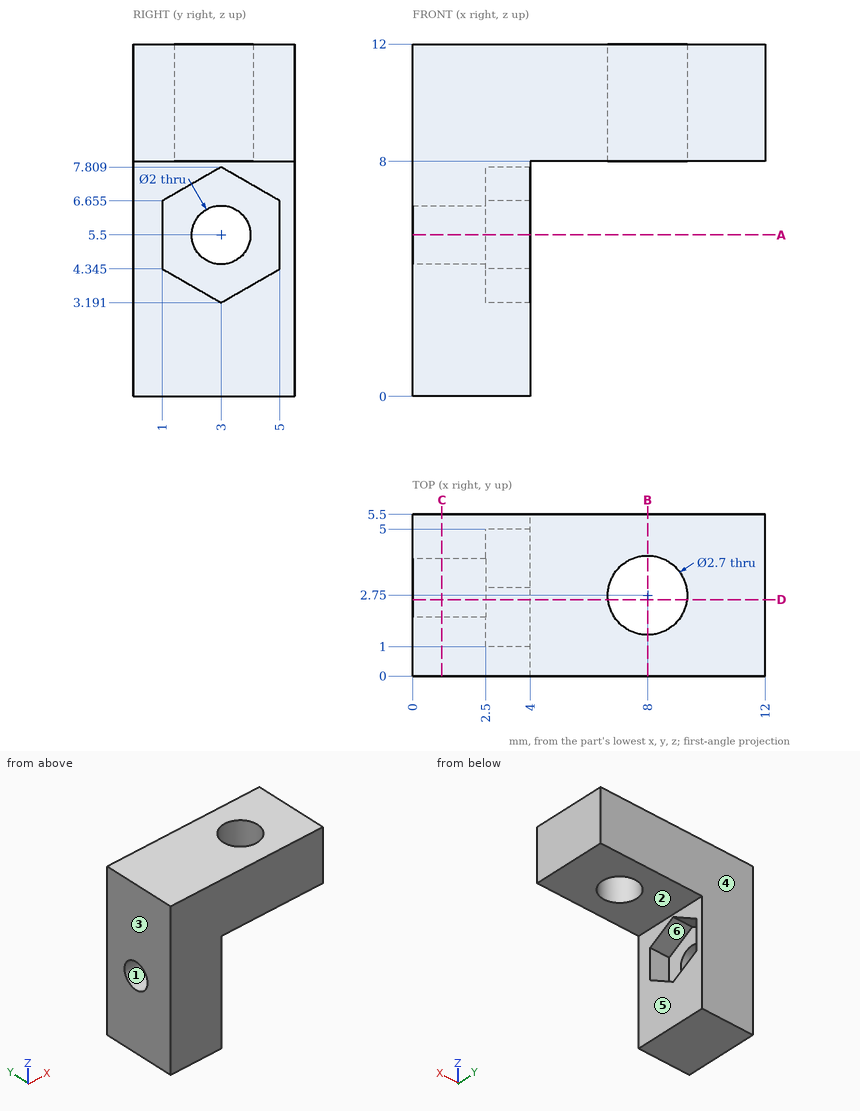
Geometry check sheet. Reference: drawing and pictorial views, mm from the part's lowest x, y, z. A direction names the side the tool comes from. Give positions to 0.01 mm unless a question says otherwise; leave off trailing zeros. Order: outer loops, then holes, each group sorted by start corner. A loop starts at its lowest first (then second) coordinate and runs counter-clockwise, first axis right, second up. Notation, with made-up numbers: M 86,25.5 L 102,25.5 A23 cw 102,48.5 Z; hole C 1.25,84 d3. An arc over 180 degrees is marked long. Use one line per item in the form item = value. Start each with the question number.
Q1. Section check B-B (x = 8). Enter the section's corners in (y, z), then the cut area to 3 significant figures.
Q2. Mould release check, pull along Z, two halves, no side actions. Record for the marked faces 1, 2 and 3: +Z half, -Z half, draft (parallel to the pull), parting line (faces both ways), or undercut.
Q3. Go/stop test with flat-tipped pins: pin 1 Ø2 at (y, z) = (3, 6.5) entering from +X; pin 2 Ø1.6 at (x, y) = (8, 2.75) entering from +Z; pin 3 Ø3 at (y, z) = (3, 2.5) entering from +X. Record where each tip stops, or that it passes through.
Q4. Section check C-C (x = 1). Enter the section's corners in (y, z).
Q5. Section check D-D (y = 2.6). Enter the section's corners in (x, z).
Q6. Section check A-A (z = 5.5). Enter the section's corners in (x, y), then the cut area to 3 significant figures.
Q7. Access from +Z, -Z, +X, -X, +Y, -Y to the whole of each face (thin tool, end or side, straight path). Record for the marked faces 4, 5 and 6.
Q8. Scan lines: line 1 along Y through (x, z) = (8, 10.6); line 2 along Y through (x, z) = (1.5, 5.5); line 3 along X through (y, z) = (4.25, 5). Record each from-to range of solid material in increasing order. Write a range as [from, to].
Evaluation:
q1.outline = M 0,8 L 1.4,8 L 1.4,12 L 0,12 Z; M 4.1,8 L 5.5,8 L 5.5,12 L 4.1,12 Z
q1.area = 11.2 mm2
q2.face_1 = undercut
q2.face_2 = -Z half
q2.face_3 = draft
q3.pin_1 = 2.5
q3.pin_2 = through
q3.pin_3 = 4
q4.outline = M 0,0 L 5.5,0 L 5.5,12 L 0,12 Z; hole C 3,5.5 d2
q5.outline = M 0,0 L 4,0 L 4,3.42 L 2.5,3.42 L 2.5,4.58 L 0,4.58 Z; M 0,6.42 L 2.5,6.42 L 2.5,7.58 L 4,7.58 L 4,8 L 6.66,8 L 6.66,12 L 0,12 Z; M 9.34,8 L 12,8 L 12,12 L 9.34,12 Z
q6.outline = M 0,0 L 4,0 L 4,1 L 2.5,1 L 2.5,2 L 0,2 Z; M 0,4 L 2.5,4 L 2.5,5 L 4,5 L 4,5.5 L 0,5.5 Z
q6.area = 11.0 mm2
q7.face_4 = +Z, -Z, +X, -X, +Y
q7.face_5 = -Z, +X, +Y, -Y
q7.face_6 = +X
q8.line_1 = [0, 1.4], [4.1, 5.5]
q8.line_2 = [0, 2], [4, 5.5]
q8.line_3 = [0, 2.5]
